Part model, mm, in its own coordinate system. A direction names the side the tool comes from. Coordinates: 2 decimals unless noted, no trailing zeros. Write each loop counter-clockwise with the first axis right and the second up, starting at its lowest first coordinate (ties: lowest second). Pieces come first, ordered by that corner, then holes. Notation, with made-up numbers: (-37, 49) -> (-2, 49) arc R28 ccw to (-2, 87) -> close; hole circle Ø5 at (-14, 8). An arc over 180 degrees is marked (long way). Write item = value, one per line. Start each with the question number.
Q1. Pin check, flat tips, straight feed: P1, Ø1, axis at x = 0.5, z = -4, coming from the +Y side; P2, Ø5, axis at y = 1, z = -5.5, coming from the +X side; P3, Ø2, axis at x = -2, z = -3.5, coming from the -Y side. Stop position of each tip, or through.
Q2. Band-saw the part on A-A, the plane y = 0. List the corners of the cut face in (x, z), plus the area to 3 significant figures.
Q3. Tool access for faces 1 (the cylindrical face through (3.233, 1.341, 3.479)), 2 (the flat face through (-2, -2, 2)), 3 (the flat face through (1.87, -3.17, -0.03)): list every direction of +Z, -Z, +X, -X, +Y, -Y with a clear straight run to the whole face (end or side of a thin tool).
Q4. Probe line 1 (Y direction, x = 0, z = 4.2); line 2 (X direction, y = -1.5, z = -3.5); line 3 (X direction, y = 0, z = -1.5). List the from-to ranges inside material, lowest first.
Q5. Band-saw the part on B-B, the plane x = 1.25. List the corners of the cut face in (y, z), plus the area to 3 significant figures.
Q6. Band-saw the part on C-C, the plane z = 1. List the corners of the cut face in (x, y) (3 decimals).
Q7. Pull direction X, two halves, no side cores. Call faces 4 (the flat face through (3.681, 0, 0)), 5 (the cylindrical face through (2.44, 0.54, 3.48)), 6 (the flat face through (-1.87, 3.17, -0.03)): released by +X, released by -X, zero draft, split by the parting line, or undercut.
Q8. Band-saw the part on D-D, the plane z = -4. List the corners of the cut face in (x, y), plus the area to 3 significant figures.
Autodesk Inventor part; units mm, degrees
ref_plane "YZ Plane" through (0, 0, 0) normal (1, 0, 0) x (0, 1, 0)
ref_plane "XZ Plane" through (0, 0, 0) normal (0, 1, 0) x (-1, 0, 0)
ref_plane "XY Plane" through (0, 0, 0) normal (0, 0, 1) x (1, 0, 0)
sketch "Sketch2" plane through (0, 0, 0) normal (0, 0, 1) x (1, 0, 0)
  line L0 (0, 4.25) -> (3.6806, 2.125)
  line L1 (3.6806, 2.125) -> (3.6806, -2.125)
  line L2 (3.6806, -2.125) -> (0, -4.25)
  line L3 (0, -4.25) -> (-3.6806, -2.125)
  line L4 (-3.6806, -2.125) -> (-3.6806, 2.125)
  line L5 (-3.6806, 2.125) -> (0, 4.25)
  point P0 (0, 0)
  point P1 (0, 0)
  point P2 (-3.6806, 0)
  dimension "d0" = 8.5
extrude "Extrusion1" add sketch "Sketch2" along normal mid plane 4
sketch "Sketch3" plane through (0, 0, 2) normal (0, 0, 1) x (1, 0, 0)
  circle A0 centre (0, 0) radius 3.5
  dimension "d3" = 7
extrude "Extrusion2" add sketch "Sketch3" along normal blind 3
sketch "Sketch4" plane through (0, 0, -2) normal (0, 0, -1) x (-1, 0, 0)
  circle A0 centre (0, 0) radius 3.5
  dimension "d6" = 7
extrude "Extrusion3" add sketch "Sketch4" along normal blind 6
sketch "Sketch5" plane through (0, 0, 5) normal (0, 0, 1) x (1, 0, 0)
  circle A0 centre (0, 0) radius 3.5
hole "Hole1" at (0, 0, 5) direction (0, 0, -1) diameter 5 depth 3
thread "Thread1"
thread "Thread2"
sketch "Sketch6" plane through (0, 0, -8) normal (0, 0, -1) x (-1, 0, 0)
  circle A0 centre (0, 0) radius 3.5
hole "Hole2" at (0, 0, -8) direction (0, 0, 1) diameter 6 depth 10
properties part number "24.1"
Ans:
q1.P1 = 3.5
q1.P2 = 3.5
q1.P3 = -3.35
q2.outline = (-3.68, -2) -> (-3.5, -2) -> (-3.5, -8) -> (-3, -8) -> (-3, 2) -> (-2.5, 2) -> (-2.5, 5) -> (-3.5, 5) -> (-3.5, 2) -> (-3.68, 2) -> close; (2.5, 2) -> (3, 2) -> (3, -8) -> (3.5, -8) -> (3.5, -2) -> (3.68, -2) -> (3.68, 2) -> (3.5, 2) -> (3.5, 5) -> (2.5, 5) -> close
q2.area = 17.4 mm2
q3.face_1 = +Z
q3.face_2 = -Z
q3.face_3 = +Z, -Z, +X, -Y
q4.line_1 = -3.5 to -2.5, 2.5 to 3.5
q4.line_2 = -3.16 to -2.6, 2.6 to 3.16
q4.line_3 = -3.68 to -3, 3 to 3.68
q5.outline = (-3.53, -2) -> (-3.27, -2) -> (-3.27, -8) -> (-2.73, -8) -> (-2.73, 2) -> (-2.17, 2) -> (-2.17, 5) -> (-3.27, 5) -> (-3.27, 2) -> (-3.53, 2) -> close; (2.17, 2) -> (2.73, 2) -> (2.73, -8) -> (3.27, -8) -> (3.27, -2) -> (3.53, -2) -> (3.53, 2) -> (3.27, 2) -> (3.27, 5) -> (2.17, 5) -> close
q5.area = 19.5 mm2
q6.outline = (-3.681, -2.125) -> (0, -4.25) -> (3.681, -2.125) -> (3.681, 2.125) -> (0, 4.25) -> (-3.681, 2.125) -> close; hole circle Ø6 at (0, 0)
q7.face_4 = released by +X
q7.face_5 = undercut
q7.face_6 = released by -X
q8.outline = circle Ø7 at (0, 0); hole circle Ø6 at (0, 0)
q8.area = 10.2 mm2
